Input: part model. Units: mm. Frame: model coordinates. Face numbers are marked on the shaded views. A direction names the side the tool comes from. Give positions to 0.01 mm unless a question says otherwise; leave off trailing zeros. Loops run counter-clockwise (first coordinate to the right, second up) from the corner with the lowest first, then second, coordinate; pieces in that order, holes last. Notation, with made-up numbers: M -25,-35 L -15,-35 A36 ccw -15,3 Z; hole C 49.25,78 d2. An arc over 180 degrees is marked long. Return JSON: item names as keys, results as strings. Group by question number.
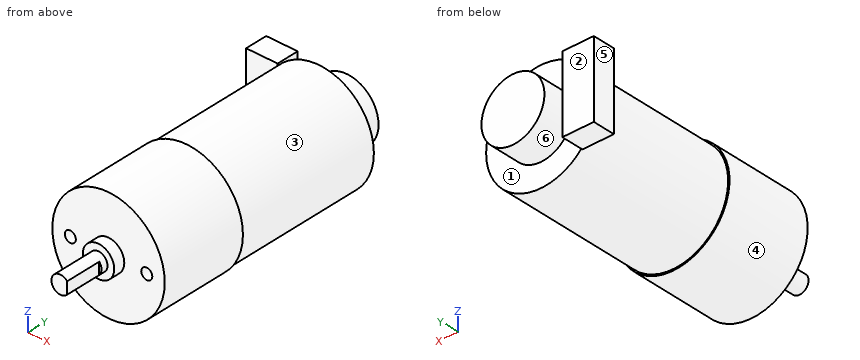
Autodesk Inventor part; units mm, degrees
ref_plane "YZ Plane" through (0, 0, 0) normal (1, 0, 0) x (0, 1, 0)
ref_plane "XZ Plane" through (0, 0, 0) normal (0, 1, 0) x (-1, 0, 0)
ref_plane "XY Plane" through (0, 0, 0) normal (0, 0, 1) x (1, 0, 0)
sketch "Schizzo1" plane through (0, 0, 0) normal (0, 1, 0) x (-1, 0, 0)
  circle A0 centre (0, 0) radius 12.2
  dimension "d0" = 24.4
extrude "Estrusione1" add sketch "Schizzo1" along normal blind 31
sketch "Schizzo2" plane through (0, 0, 0) normal (0, -1, 0) x (1, 0, 0)
  circle A0 centre (0, 0) radius 12.5
  dimension "d3" = 25
extrude "Estrusione2" add sketch "Schizzo2" along normal blind 19.5
sketch "Schizzo3" plane through (0, -19.5, 0) normal (0, -1, 0) x (1, 0, 0)
  circle A0 centre (0, 0) radius 12.2
  circle A1 centre (0, 0) radius 3.5
  dimension "d6" = 7
extrude "Estrusione3" add sketch "Schizzo3" along normal blind 2.5 contours A1
sketch "Schizzo4" plane through (0, -22, 0) normal (0, -1, 0) x (1, 0, 0)
  circle A0 centre (0, 0) radius 2
  dimension "d9" = 4
extrude "Estrusione4" add sketch "Schizzo4" along normal blind 9.5
sketch "Schizzo5" plane through (0, -31.5, 0) normal (0, -1, 0) x (1, 0, 0)
  circle A0 centre (0, 0) radius 2
  line L0 (-2, 0) -> (1.5, 0)
  line L1 (1.5, 0) -> (1.5, -1.3229)
  line L2 (1.5, 0) -> (1.5, 1.3229)
  dimension "d12" = 3.5
extrude "Estrusione5" cut sketch "Schizzo5" against normal blind 8 contours A0 L1 L2
sketch "Schizzo6" plane through (0, -19.5, 0) normal (0, -1, 0) x (1, 0, 0)
  line L0 (0, 0) -> (8.5, 0)
  circle A0 centre (8.5, 0) radius 1.5
  line L1 (8.5, 0) -> (-8.5, 0)
  line L2 (8.5, 0) -> (25.5, 0) construction
  circle A1 centre (-8.5, 0) radius 1.5
  dimension "d15" = 8.5
  dimension "d16" = 3
  dimension "d17" = 17
  dimension "d18" = 180
  dimension "d19" = 3
hole "Foro1" at (8.5, -19.5, 0) at (-8.5, -19.5, 0) direction (0, 1, 0) diameter 2.459 depth 8.8 tip angle 118
sketch "Schizzo7" plane through (0, 31, 0) normal (0, 1, 0) x (1, 0, 0)
  point P0 (0, 0)
sketch "Schizzo8" plane through (0, 31, 0) normal (0, 1, 0) x (1, 0, 0)
  circle A0 centre (0, 0) radius 7
  dimension "d30" = 14
extrude "Estrusione6" add sketch "Schizzo8" along normal blind 9 from surface at 0
sketch "Schizzo9" plane through (0, 31, 0) normal (0, 1, 0) x (1, 0, 0)
  circle A0 centre (0, 0) radius 12.2
  dimension "d31" = 24.4
extrude "Estrusione7" add sketch "Schizzo9" along normal blind 2
sketch "Schizzo10" plane through (0, 33, 0) normal (0, 1, 0) x (1, 0, 0)
  circle A0 centre (0, 0) radius 12.2
  line L0 (-12.2, 0) -> (-9.2, 0)
  line L1 (-9.2, 8.5) -> (-16.2, 8.5)
  line L2 (-16.2, 8.5) -> (-16.2, -8.5)
  line L3 (-16.2, -8.5) -> (-9.2, -8.5)
  line L4 (-9.2, -8.5) -> (-9.2, 8.5)
  dimension "d34" = 3
  dimension "d35" = 17
  dimension "d36" = 7
extrude "Estrusione8" add sketch "Schizzo10" along normal blind 5 contours L4 L0 A0 | A0 L4 L3 L2 L1 | A0 L0 L4
properties part number "7_Motore" material "M.Motore"
Item 1: Pull-direction query (X, two-part tool) for the marked faces 1, 2 and 3; classes: pulls with the +X half, pulls with the -X half, needs draft (parallel to the pull), parting line crosses it, or undercut.
Item 2: First-contact query: pin 1 Ø5 at (x, y) = (-10.5, 31.5) entering from -Z; pin 2 Ø6 at (x, y) = (5, 3) entering from +Z; pin 3 Ø3 at (x, z) = (8.5, 0) entering from -Y; pin 4 Ø5.5 at (x, z) = (1.5, 1.5) entering from -Y. Flat tips, straight axial feed; report the tip coordinate or a pass-through.
Item 3: Section C-C, the plane y = -13. Return loops of the section in (x, z).
Item 4: Reachability of the marked faces 4, 5 and 6 from +Z, -Z, +X, -X, +Y, -Y: full face, straight path, thin tool, end or side. Return the list, or none.
Item 5: Section B-B, the plane x = 0. Return loops of the section in (y, z).
Item 6: Section A-A, the plane y = 35.5. Return loops of the section in (x, z), then the cut area to 3 significant figures.
Item 7: Material intervals for line 1 (Y direction, x = 7.5, z = -1.5); line 2 (Y direction, x = 6.25, z = 0.75); line 3 (Z direction, x = 0.25, y = -17.5), sorted ascending. Write a range as from..to.
Item 8: Section D-D, the plane x = -11.25. Return loops of the section in (y, z), then the cut area to 3 significant figures.
Answer below:
{
 "1": {"face 1": "undercut", "face 2": "needs draft", "face 3": "parting line crosses it"},
 "2": {"pin 1": "z = -9.21", "pin 2": "z = 12.03", "pin 3": "y = -19.5", "pin 4": "y = -31.5"},
 "3": {"outline": "C 0,0 d25; hole C -8.5,0 d2.46; hole C 8.5,0 d2.46"},
 "4": {"face 4": "-Y", "face 5": "+Z, -Z, -X, +Y, -Y", "face 6": "+Y"},
 "5": {"outline": "M -31.5,-2 L -22,-2 L -22,-3.5 L -19.5,-3.5 L -19.5,-12.5 L 0,-12.5 L 0,-12.2 L 33,-12.2 L 33,-7 L 40,-7 L 40,7 L 33,7 L 33,12.2 L 0,12.2 L 0,12.5 L -19.5,12.5 L -19.5,3.5 L -22,3.5 L -22,2 L -31.5,2 Z"},
 "6": {"outline": "M -16.2,-8.5 L -9.2,-8.5 L -9.2,8.5 L -16.2,8.5 Z; C 0,0 d14", "area": "273 mm^2"},
 "7": {"line 1": "-19.5..33", "line 2": "-19.5..40", "line 3": "-12.5..12.5"},
 "8": {"outline": "M -19.5,-5.45 L 0,-5.45 L 0,-4.72 L 33,-4.72 L 33,-8.5 L 38,-8.5 L 38,8.5 L 33,8.5 L 33,4.72 L 0,4.72 L 0,5.45 L -19.5,5.45 Z", "area": "609 mm^2"}
}
